Read the model definition and answer for the solid it produces. Units are mm, in the model's axes. A direction names the side the tool comes from. Coordinates: 2 decimals unless noted, no trailing zeros. Order: outer loops, then holes, each group sorted by start corner. A loop starts at its lowest first (then second) coordinate and runs counter-clockwise, first axis right, second up. Notation, with made-up numbers: (77, 13) -> (112, 13) arc R14 ccw to (112, 30) -> close; hole circle Ø6 at (-27.5, 62.5). An arc over 180 degrees is marked (long way). Use CSV: the item, a comma, the result in double quotes.
```python
from build123d import *

# Parameters (mm, degrees)
SKETCH1_R            = 3.3782
BOSS_EXTRUDE1_DEPTH  = 3.175
BOSS_EXTRUDE2_DEPTH  = 4.445
SKETCH7_W            = 18.542
SKETCH7_H            = 15.24
BOSS_EXTRUDE4_DEPTH  = 8.43915
SKETCH8_R            = 1.524
CUT_EXTRUDE3_DEPTH   = 21.955
SKETCH9_R            = 10.16
CUT_EXTRUDE4_DEPTH   = 21.955
SKETCH22_W           = 6.35
SKETCH22_H           = 6.35
CUT_EXTRUDE6_DEPTH   = 9.525
SKETCH23_R           = 4.490128061
CUT_EXTRUDE7_DEPTH   = 6.35
BOSS_EXTRUDE10_DEPTH = 3.175
BOSS_EXTRUDE11_DEPTH = 3.175
SKETCH19_W           = 8.382
SKETCH19_H           = 4.445
BOSS_EXTRUDE12_DEPTH = 19.05
BOSS_EXTRUDE13_DEPTH = 4.445
CUT_EXTRUDE5_DEPTH   = 12.7


with BuildPart() as part:
    # Sketch1 → Boss-Extrude1 (new body)
    with BuildSketch(Plane(origin=(0, 0, 0), x_dir=(1, 0, 0), z_dir=(0, 1, 0))):
        with BuildLine():
            Line((0, -13.335), (25.4, -13.335))
            Line((25.4, -13.335), (25.4, 13.335))
            Line((25.4, 13.335), (0, 13.335))
            ThreePointArc((0, 13.335), (-13.335, 0), (0, -13.335))
        make_face()
        Circle(SKETCH1_R, mode=Mode.SUBTRACT)
    boss_extrude1 = extrude(amount=BOSS_EXTRUDE1_DEPTH)

    # Sketch2 → Boss-Extrude2 (add)
    with BuildSketch(Plane(origin=(0, 0, 0), x_dir=(-1, 0, 0), z_dir=(0, -1, 0))):
        Polygon((-25.4, 13.335), (-25.4, -13.335), (-13.335, -13.335), (-13.335, 0), (-13.335, 13.335), align=None)
    extrude(amount=BOSS_EXTRUDE2_DEPTH)

    # Mirror2: Boss-Extrude1 across plane
    add(boss_extrude1.mirror(Plane(origin=(0, -2.2225, 0), x_dir=(0, 0, 1), z_dir=(0, -1, 0))))

    # Sketch7 → Boss-Extrude4 (add)
    with BuildSketch(Plane(origin=(0, -7.62, 0), x_dir=(-1, 0, 0), z_dir=(0, -1, 0))):
        with Locations((-16.129, 0)):
            Rectangle(SKETCH7_W, SKETCH7_H)
    extrude(amount=BOSS_EXTRUDE4_DEPTH)

    # Sketch8 → Cut-Extrude3 (cut, through all)
    with BuildSketch(Plane(origin=(0, 0, -7.62), x_dir=(-1, 0, 0), z_dir=(0, 0, -1))):
        with Locations((-20.7645, -12.1285)):
            Circle(SKETCH8_R)
        with Locations((-11.4935, -12.1285)):
            Circle(SKETCH8_R)
    extrude(amount=-CUT_EXTRUDE3_DEPTH, mode=Mode.SUBTRACT)

    # Sketch9 → Cut-Extrude4 (cut, through all)
    with BuildSketch(Plane(origin=(0, 0, -7.62), x_dir=(-1, 0, 0), z_dir=(0, 0, -1))):
        with Locations((-16.129, -23.67915)):
            Circle(SKETCH9_R)
    extrude(amount=-CUT_EXTRUDE4_DEPTH, mode=Mode.SUBTRACT)

    # Sketch22 → Cut-Extrude6 (cut)
    with BuildSketch(Plane(origin=(0, 3.175, 0), x_dir=(1, 0, 0), z_dir=(0, 1, 0))):
        with Locations((19.3675, 0)):
            Rectangle(SKETCH22_W, SKETCH22_H)
    extrude(amount=-CUT_EXTRUDE6_DEPTH, mode=Mode.SUBTRACT)

    # Sketch23 → Cut-Extrude7 (cut)
    with BuildSketch(Plane(origin=(0, -6.35, 0), x_dir=(1, 0, 0), z_dir=(0, 1, 0))):
        with Locations((19.3675, 0)):
            Circle(SKETCH23_R)
    extrude(amount=CUT_EXTRUDE7_DEPTH, mode=Mode.SUBTRACT)

    # Sketch16 → Boss-Extrude10 (add)
    with BuildSketch(Plane(origin=(0, 3.175, 0), x_dir=(1, 0, 0), z_dir=(0, 1, 0))):
        Polygon((0, 13.335), (-13.335, 0), (-13.335, 13.335), align=None)
    extrude(amount=-BOSS_EXTRUDE10_DEPTH)

    # Sketch17 → Boss-Extrude11 (add)
    with BuildSketch(Plane.XZ.offset(7.62)):
        Polygon((-13.335, -13.335), (-13.335, 0), (0, -13.335), align=None)
    extrude(amount=-BOSS_EXTRUDE11_DEPTH)

    # Sketch19 → Boss-Extrude12 (add)
    with BuildSketch(Plane(origin=(0, 3.175, 0), x_dir=(1, 0, 0), z_dir=(0, 1, 0))):
        with Locations((-2.5019, 11.1125)):
            Rectangle(SKETCH19_W, SKETCH19_H)
    extrude(amount=BOSS_EXTRUDE12_DEPTH)

    # Sketch20 → Boss-Extrude13 (add)
    with BuildSketch(Plane.XY.offset(-8.89)):
        Polygon((-6.6929, 22.225), (-13.335, 3.175), (-6.6929, 3.175), align=None)
    extrude(amount=-BOSS_EXTRUDE13_DEPTH)

    # Sketch21 → Cut-Extrude5 (cut)
    with BuildSketch(Plane.XY.offset(-8.89)):
        Polygon((0, 20.61479766), (1.6891, 21.59), (1.6891, 18.369595321), (0, 19.34479766), align=None)
    extrude(amount=-CUT_EXTRUDE5_DEPTH, mode=Mode.SUBTRACT)


solid = part.part
```
Item 1: A tool of negligible diameter and unlimited length cuts with its end or side. For faces 4 (the flat face through (19, 0, -4)), 5 (the flat face through (0.86, 18.85, -11.08)), 6 (the flat face through (3, 0, -3)), from which of +Z, -Z, +X, -X, +Y, -Y can it reach the whole face along a straight path? Write none if from no direction.
Return value:
face 4,"none"
face 5,"+Z, -Z, +X"
face 6,"+Z, -Z, -X"
Item 2: Find section A-A, the plane x = 5. Give the vertices of the cut face in (y, z) (3 decimals), then the cut area to 3 significant figures.
Return value:
outline,"(-7.62, -13.335) -> (-4.445, -13.335) -> (-4.445, 13.335) -> (-7.62, 13.335) -> close; (0, -13.335) -> (3.175, -13.335) -> (3.175, 13.335) -> (0, 13.335) -> close"
area,"169 mm^2"
Item 3: The mould has two halves that part along X. Classify faces 1 (the flat face through (6, 3.175, 0)), 2 (the flat face through (19, 2, 3.175)), 3 (the flat face through (13.335, -2, 0)): +X half, -X half, draft (parallel to the pull), parting line (faces both ways), or undercut.
Return value:
face 1,"draft"
face 2,"undercut"
face 3,"-X half"
Item 4: Find section B-B, the plane z = 1. Give the number of separate pieces and of enclosed holes in the cut face, then the cut area to 3 significant figures.
Return value:
separate pieces,"3"
enclosed holes,"2"
area,"301 mm^2"
Item 5: Each of these flat-tipped pins is pushed along its axis until it touches: P1, Ø5.5, axis at x = 19.37, z = 0, coming from the -Y side; P2, Ø4, axis at x = 18, y = -10, coming from the -Z side; P3, Ø1.3, axis at y = -1.5, z = -2, coming from the -X side (3 decimals). Where does it stop, or does it pass through?
Return value:
P1,"stops at y = -15.47"
P2,"stops at z = -7.62"
P3,"stops at x = 13.335"
Item 6: Straight lines are drawn through the part: line 1 along X through (y, z) = (-12, -2.5); line 2 along X through (y, z) = (-4.75, 0) (3 decimals); line 3 along Z through (x, y) = (0, 1) (3 decimals). For each, find the intervals that lie inside material, in ascending order.
Return value:
line 1,"x = 6.86 to 9.97, 13.01 to 19.25, 22.28 to 25.4"
line 2,"x = -13.335 to -3.378, 3.378 to 14.877, 23.858 to 25.4"
line 3,"z = -13.335 to -3.378, 3.378 to 13.335"
Item 7: Find section C-C, the plane y = 1. Give the vertices of the cut face in (x, z) (1 decimal).
Return value:
outline,"(-13.3, -13.3) -> (25.4, -13.3) -> (25.4, 13.3) -> (0, 13.3) arc R13.3 ccw to (-13.3, 0) -> close; hole circle Ø6.8 at (0, 0); hole (16.2, -3.2) -> (22.5, -3.2) -> (22.5, 3.2) -> (16.2, 3.2) -> close"
Item 8: Find section D-D, the plane x = -2.5. Give the vertices of the cut face in (y, z) (3 decimals).
Return value:
outline,"(-7.62, -13.335) -> (-4.445, -13.335) -> (-4.445, -2.272) -> (-7.62, -2.272) -> close; (-7.62, 2.272) -> (-4.445, 2.272) -> (-4.445, 13.099) -> (-7.62, 13.099) -> close; (0, -13.335) -> (22.225, -13.335) -> (22.225, -8.89) -> (3.175, -8.89) -> (3.175, -2.272) -> (0, -2.272) -> close; (0, 2.272) -> (3.175, 2.272) -> (3.175, 13.099) -> (0, 13.099) -> close"
